Source: three-view drawing plus pictorial views. Frame: mm from the lowest corner of the part. A direction names the side the tool comes from. Round coordinates to 2 decimals unless told otherwise and drop trailing zeros. Write each loop counter-clockwise with the first axis right and the second up, starting at its lowest first coordinate (ties: lowest second). Pieces come first, ordered by that corner, then holes. Notation, with made-up numbers: M 39,28.25 L 71,28.25 A19 cw 71,32.25 Z; hole C -9,-20.5 d3. An arc over 180 degrees is marked long. Answer as CSV lines item,"result". Start each with the question number.
Q1. Ray query, probe 1 along X at (y, z) = (25.75, 53); probe 2 along Y at (x, z) = (230, 106). Return the intervals inside material, ascending.
Q2. First-contact query: pin 1 (5 mm diameter, centred on y = 14.5, z = 45.5, fed in from -X); pin 2 (1.5 mm diameter, centred on y = 10, z = 65, fed in from +X); pin 3 (20 mm diameter, centred on x = 236, z = 111.5, fed in from -Y). Flat tips, straight axial feed; report the tip coordinate or a pass-through.
Q3. Section query A-A on z = 93. Output: boundary loops of the cut face in (x, y), and give its area (3 significant figures).
Q4. Reachability of the marked faces 1 and 2 from +Z, -Z, +X, -X, +Y, -Y: full face, straight path, thin tool, end or side. Return the list, or none.
Q5. Section query B-B on y = 6. Output: boundary loops of the cut face in (x, z).
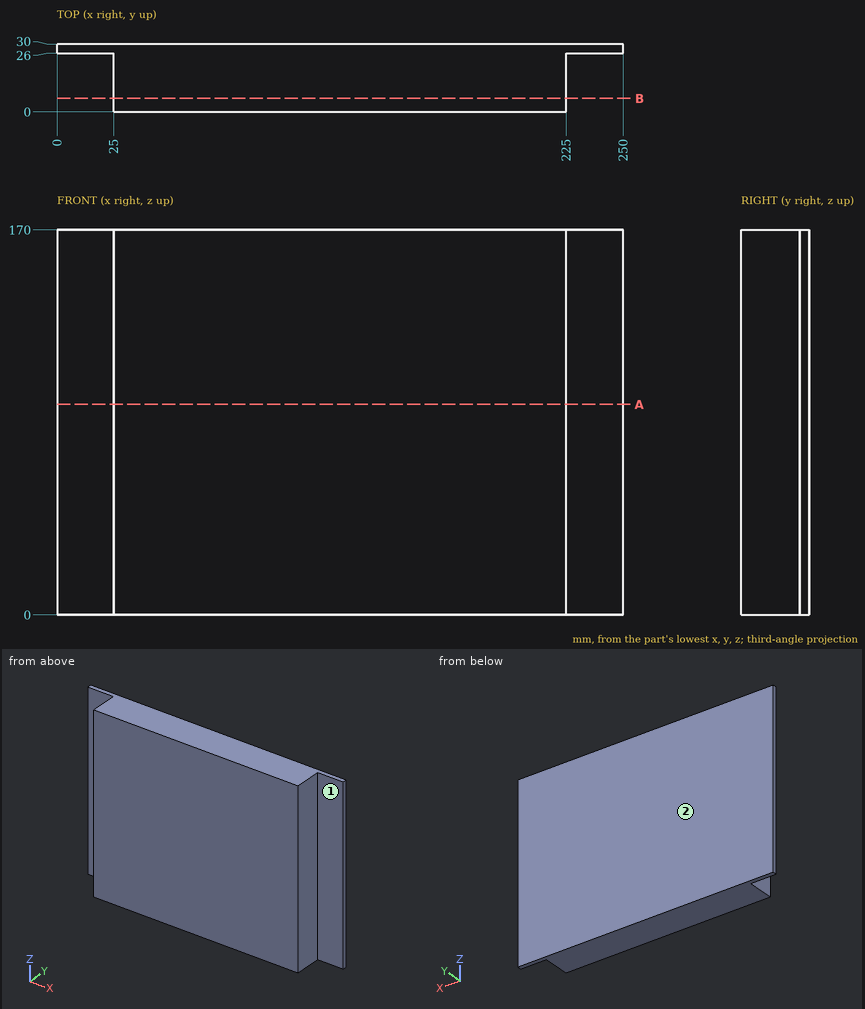
Entries:
1,probe 1,"x = 25 to 225"
1,probe 2,"y = 26 to 30"
2,pin 1,"stops at x = 25"
2,pin 2,"stops at x = 225"
2,pin 3,"stops at y = 26"
3,outline,"M 0,26 L 25,26 L 25,0 L 225,0 L 225,26 L 250,26 L 250,30 L 0,30 Z"
3,area,"6,200 mm^2"
4,face 1,"+Z, -Z, +X, -Y"
4,face 2,"+Z, -Z, +X, -X, +Y"
5,outline,"M 25,0 L 225,0 L 225,170 L 25,170 Z"
